The listing builds one solid part. Answer for the finished solid, in the listing's coordinates (mm). A direction names the side the tool comes from. Coordinates: 2 decimals unless noted, no trailing zeros. Order: outer loops, then holes, each group sorted by start corner. A loop starts at its lowest first (then second) coordinate and runs counter-clockwise, first axis right, second up. Notation, with made-up numbers: (-7.75, 85.25) -> (8.25, 85.25) arc R18 ccw to (8.25, 106.25) -> close; hole circle Ø10 at (45.5, 35). An arc over 180 degrees is marked (long way). Write item = value, one per line. Start each with the question number.
```python
from build123d import *

# Parameters (mm, degrees)
SKETCH1_W           = 45
SKETCH1_H           = 54
SKETCH1_W_2         = 40
SKETCH1_H_2         = 49
BOSS_EXTRUDE1_DEPTH = 13.3
SKETCH3_W           = 45
SKETCH3_H           = 54
BOSS_EXTRUDE2_DEPTH = 2.5
BOSS_EXTRUDE4_DEPTH = 13.3
SKETCH5_W           = 11
SKETCH5_H           = 30
CUT_EXTRUDE1_DEPTH  = 5
SKETCH6_W           = 12
SKETCH6_H           = 6
CUT_EXTRUDE2_DEPTH  = 5
SKETCH7_R           = 1.456693422
SKETCH7_R_2         = 1.2474688
SKETCH7_W           = 8.87889324
SKETCH7_H           = 5.133110155
BOSS_EXTRUDE5_DEPTH = 7.3
FILLET1_R           = 1
CUT_EXTRUDE3_DEPTH  = 7.3
FILLET2_R           = 1
CHAMFER2_SIZE       = 1.25
CHAMFER3_SIZE       = 1.25
CHAMFER4_SIZE       = 1.25
SKETCH9_W           = 21.210465444
SKETCH9_H           = 4.165192571
BOSS_EXTRUDE6_DEPTH = 13.3
SKETCH10_R          = 1
CUT_EXTRUDE4_DEPTH  = 7.3
SKETCH11_R          = 1.25
CUT_EXTRUDE5_DEPTH  = 10


with BuildPart() as part:
    # Sketch1 → Boss-Extrude1 (new body)
    with BuildSketch(Plane(origin=(0, 0, 0), x_dir=(1, 0, 0), z_dir=(0, 1, 0))):
        Rectangle(SKETCH1_W, SKETCH1_H)
        Rectangle(SKETCH1_W_2, SKETCH1_H_2, mode=Mode.SUBTRACT)
    extrude(amount=BOSS_EXTRUDE1_DEPTH)

    # Sketch3 → Boss-Extrude2 (add)
    with BuildSketch(Plane.XZ):
        Rectangle(SKETCH3_W, SKETCH3_H)
    extrude(amount=BOSS_EXTRUDE2_DEPTH)

    # Sketch4 → Boss-Extrude4 (add, through all)
    with BuildSketch(Plane(origin=(0, 0, 0), x_dir=(1, 0, 0), z_dir=(0, 1, 0))):
        Polygon((-12.65, -16.7), (-10.15, -19.2), (-10.15, -24.5), (-20, -24.5), (-20, -16.7), align=None)
        Polygon((12.65, -16.7), (10.15, -19.2), (10.15, -24.5), (20, -24.5), (20, -16.7), align=None)
    extrude(amount=BOSS_EXTRUDE4_DEPTH)

    # Sketch5 → Cut-Extrude1 (cut)
    with BuildSketch(Plane.XZ.offset(2.5)):
        with Locations((-13.3, -5.33)):
            Rectangle(SKETCH5_W, SKETCH5_H)
    extrude(amount=-CUT_EXTRUDE1_DEPTH, mode=Mode.SUBTRACT)

    # Sketch6 → Cut-Extrude2 (cut)
    with BuildSketch(Plane(origin=(22.5, 0, 0), x_dir=(0, 0, -1), z_dir=(1, 0, 0))):
        with Locations((8.5, 5.8)):
            Rectangle(SKETCH6_W, SKETCH6_H)
    extrude(amount=-CUT_EXTRUDE2_DEPTH, mode=Mode.SUBTRACT)

    # Sketch7 → Boss-Extrude5 (add)
    with BuildSketch(Plane(origin=(0, 0, 0), x_dir=(1, 0, 0), z_dir=(0, 1, 0))):
        with Locations(Location((4.5, 18.5, 0), (0, 0, 90))):
            Circle(SKETCH7_R)
        with Locations(Location((-12, -12.183033551, 0), (0, 0, 90))):
            Circle(SKETCH7_R_2)
        with Locations((0, -18.659549076)):
            Rectangle(SKETCH7_W, SKETCH7_H)
    extrude(amount=BOSS_EXTRUDE5_DEPTH)

    # Fillet1
    fillet1_edges = [part.edges().sort_by_distance(p)[0] for p in [
        (-22.5, -2.5, 0),
        (0, -2.5, -27),
        (22.5, -2.5, 0),
        (0, -2.5, 27),
        (-22.5, 5.4, -27),
        (22.5, 5.4, -27),
        (22.5, 5.4, 27),
        (-22.5, 5.4, 27),
    ]]
    fillet(fillet1_edges, radius=FILLET1_R)

    # Sketch8 → Cut-Extrude3 (cut)
    with BuildSketch(Plane(origin=(0, 0, 0), x_dir=(1, 0, 0), z_dir=(0, 1, 0))):
        with BuildLine():
            Line((-3.329584965, 14.5), (14.775033283, 14.5))
            ThreePointArc((14.775033283, 14.5), (16.275033283, 13), (14.775033283, 11.5))
            Line((14.775033283, 11.5), (-3.329584965, 11.5))
            ThreePointArc((-3.329584965, 11.5), (-4.829584965, 13), (-3.329584965, 14.5))
        make_face()
        with BuildLine():
            Line((-3.329584965, 8.5), (14.775033283, 8.5))
            ThreePointArc((14.775033283, 8.5), (16.275033283, 7), (14.775033283, 5.5))
            Line((14.775033283, 5.5), (-3.329584965, 5.5))
            ThreePointArc((-3.329584965, 5.5), (-4.829584965, 7), (-3.329584965, 8.5))
        make_face()
        with BuildLine():
            Line((-3.329584965, 2.5), (14.775033283, 2.5))
            ThreePointArc((14.775033283, 2.5), (16.275033283, 1), (14.775033283, -0.5))
            Line((14.775033283, -0.5), (-3.329584965, -0.5))
            ThreePointArc((-3.329584965, -0.5), (-4.829584965, 1), (-3.329584965, 2.5))
        make_face()
        with BuildLine():
            Line((-3.329584965, -3.5), (14.775033283, -3.5))
            ThreePointArc((14.775033283, -3.5), (16.275033283, -5), (14.775033283, -6.5))
            Line((14.775033283, -6.5), (-3.329584965, -6.5))
            ThreePointArc((-3.329584965, -6.5), (-4.829584965, -5), (-3.329584965, -3.5))
        make_face()
        with BuildLine():
            Line((-3.329584965, -9.5), (14.775033283, -9.5))
            ThreePointArc((14.775033283, -9.5), (16.275033283, -11), (14.775033283, -12.5))
            Line((14.775033283, -12.5), (-3.329584965, -12.5))
            ThreePointArc((-3.329584965, -12.5), (-4.829584965, -11), (-3.329584965, -9.5))
        make_face()
    extrude(amount=-CUT_EXTRUDE3_DEPTH, mode=Mode.SUBTRACT)

    # Fillet2
    fillet2_edges = [part.edges().sort_by_distance(p)[0] for p in [
        (-4.43944662, 0, 18.659549076),
        (0, 0, 21.226104153),
        (4.43944662, 0, 18.659549076),
        (0, 0, 16.092993998),
        (4.5, 0, -17.043306578),
        (-12, 0, 13.430502351),
    ]]
    fillet(fillet2_edges, radius=FILLET2_R)

    # Chamfer2
    chamfer2_edges = [part.edges().sort_by_distance(p)[0] for p in [
        (5.722724159, -2.5, -11.5),
        (16.275033283, -2.5, -13),
        (5.722724159, -2.5, -14.5),
        (-4.829584965, -2.5, -13),
        (5.722724159, -2.5, -5.5),
        (16.275033283, -2.5, -7),
        (5.722724159, -2.5, -8.5),
        (-4.829584965, -2.5, -7),
        (5.722724159, -2.5, 0.5),
        (16.275033283, -2.5, -1),
        (5.722724159, -2.5, -2.5),
        (-4.829584965, -2.5, -1),
        (5.722724159, -2.5, 6.5),
        (16.275033283, -2.5, 5),
        (5.722724159, -2.5, 3.5),
        (-4.829584965, -2.5, 5),
        (5.722724159, -2.5, 12.5),
        (16.275033283, -2.5, 11),
        (5.722724159, -2.5, 9.5),
        (-4.829584965, -2.5, 11),
    ]]
    chamfer(chamfer2_edges, length=CHAMFER2_SIZE)

    # Chamfer3
    chamfer3_edges = [part.edges().sort_by_distance(p)[0] for p in [
        (5.722724159, 0, 12.5),
        (16.275033283, 0, 11),
        (-4.829584965, 0, 11),
        (5.722724159, 0, 9.5),
        (5.722724159, 0, 6.5),
        (16.275033283, 0, 5),
        (-4.829584965, 0, 5),
        (5.722724159, 0, 3.5),
        (5.722724159, 0, 0.5),
        (16.275033283, 0, -1),
        (-4.829584965, 0, -1),
        (5.722724159, 0, -2.5),
        (5.722724159, 0, -5.5),
        (16.275033283, 0, -7),
        (-4.829584965, 0, -7),
        (5.722724159, 0, -8.5),
        (5.722724159, 0, -11.5),
        (16.275033283, 0, -13),
        (-4.829584965, 0, -13),
        (5.722724159, 0, -14.5),
    ]]
    chamfer(chamfer3_edges, length=CHAMFER3_SIZE - 0.0001)  # a hair under: the kernel refuses the full size

    # Chamfer4
    chamfer4_edges = [part.edges().sort_by_distance(p)[0] for p in [
        (-18.8, -2.5, -5.33),
        (-13.3, -2.5, -20.33),
        (-7.8, -2.5, -5.33),
        (-13.3, -2.5, 9.67),
    ]]
    chamfer(chamfer4_edges, length=CHAMFER4_SIZE)

    # Sketch9 → Boss-Extrude6 (add, through all)
    with BuildSketch(Plane(origin=(0, 0, 0), x_dir=(1, 0, 0), z_dir=(0, 1, 0))):
        with Locations((-9.394767278, 22.417403715)):
            Rectangle(SKETCH9_W, SKETCH9_H)
    extrude(amount=BOSS_EXTRUDE6_DEPTH)

    # Sketch10 → Cut-Extrude4 (cut)
    with BuildSketch(Plane(origin=(0, 13.3, 0), x_dir=(1, 0, 0), z_dir=(0, 1, 0))):
        with Locations(Location((-10.018444645, 23.665, 0), (0, 0, 270))):
            Circle(SKETCH10_R)
        with Locations(Location((-17, -22, 0), (0, 0, 270))):
            Circle(SKETCH10_R)
        with Locations(Location((17, -22, 0), (0, 0, 270))):
            Circle(SKETCH10_R)
    extrude(amount=-CUT_EXTRUDE4_DEPTH, mode=Mode.SUBTRACT)

    # Sketch11 → Cut-Extrude5 (cut)
    with BuildSketch(Plane(origin=(0, 0, -27), x_dir=(-1, 0, 0), z_dir=(0, 0, -1))):
        with Locations((-12.75, 3.25)):
            Circle(SKETCH11_R)
    extrude(amount=-CUT_EXTRUDE5_DEPTH, mode=Mode.SUBTRACT)


solid = part.part
```
Item 1: Section B-B, the plane z = -18.5 is taken. Give the vertices of the cut face in (x, y), then the cut area to 3 significant figures.
Item 2: Section D-D, the plane y = 11.25 is taken. Give the vertices of the cut face in (x, z) (3 decimals), then the cut area to 3 significant figures.
Item 3: Consider probe 1 along X at (y, z) = (8, 22); probe 2 along X at (y, z) = (12.5, 3); probe 3 along Y at (x, z) = (12.75, -25.9). Determine where each line is inside the solid, lowest interval first.
Item 4: Section A-A, the plane z = -7 is taken. Give the number of separate pieces and of enclosed holes in the cut face, then the cut area to 3 significant figures.
Item 5: Which of the six approach directions +Z, -Z, +X, -X, +Y, -Y give full straight-line access (tool end or side, diameter ignored) to faces 3 (the conical face through (-5.05, -1.47, 4.96)), 4 (the flat face through (10, 7, -24.5)), 5 (the flat face through (-13, -1, -20.33)), 6 (the flat face through (0, 6, -27))?
Item 6: Each of these flat-tipped pins is pushed along its axis until it touches: pin 1 (1 mm diameter, centred on x = -10, z = -24, fed in from +Y); pin 2 (5.5 mm diameter, centred on x = -1.5, z = 19.5, fed in from +Y); pin 3 (4 mm diameter, centred on y = 6, z = -7, fed in from +X). Where does it stop, or does it pass through?
Item 7: For a pull along X with two mould halves and no side action, classify faces 1 (the flat face through (-10, -2.5, 12)), 2 (the conical face through (16.492, -1.467, 5.038)) as pulls with the +X half, pulls with the -X half, needs draft (parallel to the pull), parting line crosses it, or undercut.
A:
q1.outline = (-22.5, -1.5) arc R1 ccw to (-21.5, -2.5) -> (-20.05, -2.5) -> (-18.8, -1.25) -> (-18.8, 0) -> (-20, 0) -> (-20, 13.3) -> (-22.5, 13.3) -> close; (-7.8, -1.25) -> (-6.55, -2.5) -> (21.5, -2.5) arc R1 ccw to (22.5, -1.5) -> (22.5, 13.3) -> (20, 13.3) -> (20, 0) -> (6.96, 0) arc R1 cw to (5.96, 1) -> (5.96, 7.3) -> (3.04, 7.3) -> (3.04, 1) arc R1 cw to (2.04, 0) -> (-7.8, 0) -> close
q1.area = 171 mm^2
q2.outline = (-22.5, -26) arc R1 ccw to (-21.5, -27) -> (21.5, -27) arc R1 ccw to (22.5, -26) -> (22.5, 26) arc R1 ccw to (21.5, 27) -> (-21.5, 27) arc R1 ccw to (-22.5, 26) -> close; hole (-20, -20.335) -> (1.21, -20.335) -> (1.21, -24.5) -> (20, -24.5) -> (20, 16.7) -> (12.65, 16.7) -> (10.15, 19.2) -> (10.15, 24.5) -> (-10.15, 24.5) -> (-10.15, 19.2) -> (-12.65, 16.7) -> (-20, 16.7) -> close; hole circle Ø2 at (-17, 22); hole circle Ø2 at (-10.018, -23.665); hole circle Ø2 at (17, 22)
q2.area = 695 mm^2
q3.probe_1 = -22.5 to -18, -16 to -10.15, 10.15 to 16, 18 to 22.5
q3.probe_2 = -22.5 to -20, 20 to 22.5
q3.probe_3 = -2.5 to 2, 4.5 to 13.3
q4.separate_pieces = 4
q4.enclosed_holes = 0
q4.area = 78.6 mm^2
q5.face_3 = -Y
q5.face_4 = +Y
q5.face_5 = +Y, -Y
q5.face_6 = -Z, +X, -X, +Y, -Y
q6.pin_1 = 6
q6.pin_2 = 7.3
q6.pin_3 = -20
q7.face_1 = needs draft
q7.face_2 = undercut
